```python
from build123d import *

# Parameters (mm, degrees)
SKETCH1_R           = 16.9
BOSS_EXTRUDE1_DEPTH = 19
SKETCH2_R           = 4.5
CUT_EXTRUDE2_DEPTH  = 38
CUT_EXTRUDE3_DEPTH  = 10
CUT_EXTRUDE4_DEPTH  = 4


with BuildPart() as part:
    # Sketch1 → Boss-Extrude1 (new, symmetric)
    with BuildSketch(Plane.XY):
        with BuildLine():
            Line((47, -69.313412318), (47, -39.313412318))
            Line((47, -39.313412318), (26.457513111, -39.313412318))
            ThreePointArc((26.457513111, -39.313412318), (25.35270378, -37.792402472), (24.27668208, -36.250892852))
            Line((24.27668208, -36.250892852), (10.123257354, 98.409948263))
            ThreePointArc((10.123257354, 98.409948263), (11.210647408, 108.042873382), (16.25, 116.324213184))
            ThreePointArc((16.25, 116.324213184), (0, 154.386587682), (-16.25, 116.324213184))
            ThreePointArc((-16.25, 116.324213184), (-11.210647408, 108.042873382), (-10.123257354, 98.409948263))
            Line((-10.123257354, 98.409948263), (-24.27668208, -36.250892852))
            ThreePointArc((-24.27668208, -36.250892852), (-25.35270378, -37.792402472), (-26.457513111, -39.313412318))
            Line((-26.457513111, -39.313412318), (-47, -39.313412318))
            Line((-47, -39.313412318), (-47, -69.313412318))
            Line((-47, -69.313412318), (-40, -69.313412318))
            Line((-40, -69.313412318), (-27, -69.313412318))
            ThreePointArc((-27, -69.313412318), (0, -42.313412318), (27, -69.313412318))
            Line((27, -69.313412318), (40, -69.313412318))
            Line((40, -69.313412318), (47, -69.313412318))
        make_face()
        with Locations((0, 131.886587682)):
            Circle(SKETCH1_R, mode=Mode.SUBTRACT)
    extrude(amount=BOSS_EXTRUDE1_DEPTH, both=True)

    # Sketch2 → Cut-Extrude2 (cut)
    with BuildSketch(Plane.XZ.offset(69.313412318)):
        with BuildLine():
            Line((-38, 19), (-47, 19))
            Line((-47, 19), (-47, 6.6e-08))
            ThreePointArc((-47, 6.6e-08), (-44.363961007, 6.363961054), (-38, 9))
            Line((-38, 9), (-38, 19))
        make_face()
        with BuildLine():
            ThreePointArc((-38, -9), (-44.363961054, -6.363961007), (-47, 6.6e-08))
            Line((-47, 6.6e-08), (-47, -19))
            Line((-47, -19), (-38, -19))
            Line((-38, -19), (-38, -9))
        make_face()
        with BuildLine():
            Line((47, 19), (38, 19))
            Line((38, 19), (38, 9))
            ThreePointArc((38, 9), (44.363961031, 6.363961031), (47, 0))
            Line((47, 0), (47, 19))
        make_face()
        with BuildLine():
            Line((38, -9), (38, -19))
            Line((38, -19), (47, -19))
            Line((47, -19), (47, 0))
            ThreePointArc((47, 0), (44.363961031, -6.363961031), (38, -9))
        make_face()
        with Locations(Location((38, 0, 0), (0, 0, 270))):
            Circle(SKETCH2_R)
        with Locations(Location((-38, 0, 0), (0, 0, 270))):
            Circle(SKETCH2_R)
    extrude(amount=-CUT_EXTRUDE2_DEPTH, mode=Mode.SUBTRACT)

    # Sketch3 → Cut-Extrude3 (cut)
    with BuildSketch(Plane.XY.offset(19)):
        with BuildLine():
            Line((-26.457513111, -39.313412318), (-22.5, 131.886587682))
            ThreePointArc((-22.5, 131.886587682), (0, 109.386587682), (22.5, 131.886587682))
            Line((22.5, 131.886587682), (26.457513111, -39.313412318))
            ThreePointArc((26.457513111, -39.313412318), (0, -29.313412318), (-26.457513111, -39.313412318))
        make_face()
    cut_extrude3 = extrude(amount=-CUT_EXTRUDE3_DEPTH, mode=Mode.SUBTRACT)

    # Mirror1: Cut-Extrude3 across plane
    add(cut_extrude3.mirror(Plane.XY), mode=Mode.SUBTRACT)

    # Sketch4 → Cut-Extrude4 (cut)
    with BuildSketch(Plane.XY.offset(9)):
        with BuildLine():
            Line((8, 76.286587682), (8, -13.713412318))
            ThreePointArc((8, -13.713412318), (0, -21.713412318), (-8, -13.713412318))
            Line((-8, -13.713412318), (-8, 76.286587682))
            ThreePointArc((-8, 76.286587682), (0, 84.286587682), (8, 76.286587682))
        make_face()
    cut_extrude4 = extrude(amount=-CUT_EXTRUDE4_DEPTH, mode=Mode.SUBTRACT)

    # Mirror2: Cut-Extrude4 across plane
    add(cut_extrude4.mirror(Plane.XY), mode=Mode.SUBTRACT)


solid = part.part
```
Can you work these out from the model? Positions are in its coordinate system, mm. A direction names the side the tool comes from. Coordinates: 2 decimals unless noted, no trailing zeros. Loops run counter-clockwise (first coordinate to the right, second up) from the corner with the lowest first, then second, coordinate; pieces in that order, holes last.
1) Imagine slicing it at D-D on x = -35.5. List the corners of the cut face in (y, z) for me, plus the area to 4 significant figures.
2) Thinking about a two-plate mould opening in Y: for faces 5 (the cylindrical face through (-42.39, -54.52, 0.98)), 6 (the flat face through (0, 32, 5)), 7 (the flat face through (-33, -69.313, 0)), 8 (the flat face through (-32, -39.313, 0)), which applies, pulls with the +Y half, pulls with the -Y half, needs draft (parallel to the pull), parting line crosses it, or undercut?
3) I need wall thicknesses on probe 1 along Y at (x, z) = (0.5, -8); probe 2 along Y at (x, z) = (6, -11.5); probe 3 along Z at (x, y) = (-2, -17). Which ranges of each line are inside material? Lowest first, please.
4) For pin 1 (8 mm diameter, centred on x = 13.5, z = 7, fed in from -Y); pin 2 (5 mm diameter, centred on x = 17, y = 51.5, fed in from -Z); pin 3 (3 mm diameter, centred on y = -58.5, z = 15.5, fed in from -X); pin 4 (7 mm diameter, centred on x = 38, z = 0, fed in from +Y), each with a flat end and sliding along its axis, tell me the tip position at first contact or that it passes through.
5) Which directions (+Z, -Z, +X, -X, +Y, -Y) give clear straight access to the entire face, cutting with the end or side of a thin tool? Please do faces 1 (the cylindrical face through (0.18, -21.71, -7.03)), 2 (the flat face through (-8, 31, 7)), 3 (the cylindrical face through (-3.664, 115.388, -0.266)), 4 (the flat face through (-17.1, 32.02, 0.13)).
6) Imagine slicing it at A-A on x = 0. List the corners of the cut face in (y, z) for me, plus the area to 3 significant figures.
7) Imagine slicing it at B-B on x = -13. List the corners of the cut face in (y, z) for me, plus the area to 3 significant figures.
8) Imagine slicing it at C-C on y = 67. List the corners of the cut face in (x, z) for me.
Completed:
1. outline: (-69.31, -19) - (-39.31, -19) - (-39.31, -3.74) - (-69.31, -3.74) - close; (-69.31, 3.74) - (-39.31, 3.74) - (-39.31, 19) - (-69.31, 19) - close
1. area: 915.5 mm2
2. face 5: needs draft
2. face 6: undercut
2. face 7: pulls with the -Y half
2. face 8: pulls with the +Y half
3. probe 1: y = -42.32 to -21.7, 84.27 to 114.99, 148.78 to 154.38
3. probe 2: y = -42.99 to -29.77, 110.2 to 116.09, 147.69 to 153.57
3. probe 3: z = -5 to 5
4. pin 1: stops at y = -48.75
4. pin 2: stops at z = -9
4. pin 3: stops at x = -38
4. pin 4: passes through
5. face 1: -Z
5. face 2: +Z
5. face 3: +Z, -Z
5. face 4: +Z, -Z, -X
6. outline: (-42.31, -19) - (-29.31, -19) - (-29.31, -9) - (-21.71, -9) - (-21.71, -5) - (84.29, -5) - (84.29, -9) - (109.39, -9) - (109.39, -19) - (114.99, -19) - (114.99, 19) - (109.39, 19) - (109.39, 9) - (84.29, 9) - (84.29, 5) - (-21.71, 5) - (-21.71, 9) - (-29.31, 9) - (-29.31, 19) - (-42.31, 19) - close; (148.79, -19) - (154.39, -19) - (154.39, 19) - (148.79, 19) - close
6. area: 2,570 mm2
7. outline: (-45.65, -19) - (-31.48, -19) - (-31.48, -9) - (71.04, -9) - (71.04, 9) - (-31.48, 9) - (-31.48, 19) - (-45.65, 19) - close; (111.99, -9) - (113.52, -9) - (113.52, -19) - (121.09, -19) - (121.09, 19) - (113.52, 19) - (113.52, 9) - (111.99, 9) - close; (142.69, -19) - (150.25, -19) - (150.25, 19) - (142.69, 19) - close
7. area: 2,990 mm2
8. outline: (-13.42, -9) - (-8, -9) - (-8, -5) - (8, -5) - (8, -9) - (13.42, -9) - (13.42, 9) - (8, 9) - (8, 5) - (-8, 5) - (-8, 9) - (-13.42, 9) - close
